Here's how the part is built. I have some questions about the finished solid (model axes, mm). Face numbers are marked on the shaded views. Coordinates: 2 decimals unless noted, no trailing zeros. Loops run counter-clockwise (first coordinate to the right, second up) from the corner with the lowest first, then second, coordinate; pieces in that order, holes last. Notation, with made-up numbers: M 33,36.25 L 67,36.25 A27 ccw 67,55.25 Z; hole C 62,25.25 d7. An arc over 180 degrees is marked long. Use CSV: the item, a comma, the result in double quotes. Start each with the question number.
Q1. For pin 1 Ø8 at (x, y) = (-20.5, 55.5) entering from -Z; pin 2 Ø10.5 at (x, z) = (-53, -18.5) entering from -Y; pin 3 Ø3 at (x, y) = (-41, 46) entering from +Z; pin 4 Ø3 at (x, z) = (-47, 41.5) entering from -Y, each with a flat end and sliding along its axis, tell me the tip position at first contact or that it passes through.
Q2. If we section it at C-C (z = 44): Please give me the cut outline in (x, y).
Q3. If we section it at B-B (x = -44): State how many separate pieces and enclosed holes the cut face has, and give its area (3 significant figures).
Q4. If we mould it in two halves opening along Z, with no side actions, what happens to the marked faces 1, 2, 3 and 4? For each: +Z half, -Z half, draft (parallel to the pull), parting line (faces both ways), or undercut.
Q5. If we section it at A-A (z = 68): Please give me the cut outline in (x, y).
Q6. Please list where these lines run through material, in increasing order: probe 1 along Y at (x, z) = (-40, 65); probe 2 along X at (y, z) = (7, 12); probe 3 along Z at (x, y) = (-22.5, 64). Write a range as [from, to].
Q7. If we section it at D-D (y = 53): Please give me the cut outline in (x, z).
from build123d import *

# Parameters (mm, degrees)
F0_W      = 76
F0_H      = 76
F0_W_2    = 68
F0_H_2    = 68
F1_DEPTH  = 100
F2_W      = 68
F2_H      = 4
F3_DEPTH  = 25
F5_DEPTH  = 72
F7_DEPTH  = 76
F9_DEPTH  = 25
F11_DEPTH = 72


with BuildPart() as f1:
    # F0 (on Top) → F1 (new body)
    with BuildSketch(Plane.XY):
        with Locations((-38, 38)):
            Rectangle(F0_W, F0_H)
        with Locations((-38, 38)):
            Rectangle(F0_W_2, F0_H_2, mode=Mode.SUBTRACT)
    extrude(amount=F1_DEPTH)

    # F2 (on face) → F3 (join)
    with BuildSketch(Plane.XY):
        Polygon((-76, 76), (-76, 0), (-72, 0), (-72, 72), (-72, 76), align=None)
        with Locations((-38, 74)):
            Rectangle(F2_W, F2_H)
        Polygon((-4, 76), (-4, 72), (-4, 0), (0, 0), (0, 76), align=None)
    extrude(amount=-F3_DEPTH)

    # F4 (on face) → F5 (join, through all)
    with BuildSketch(Plane(origin=(-76, 0, 0), x_dir=(0, -1, 0), z_dir=(-1, 0, 0))):
        Polygon((-10.85203, -25), (-71.971662, 0), (-76, 0), (-76, -2.726357), (-21.37715, -25), align=None)
    extrude(amount=-F5_DEPTH)

    # F6 (on face) → F7 (cut, through all)
    with BuildSketch(Plane(origin=(-76, 0, 0), x_dir=(0, -1, 0), z_dir=(-1, 0, 0))):
        with BuildLine():
            Line((0, -25), (0, 0))
            ThreePointArc((0, 0), (-9.849808, -7.286393), (-12.617335, -19.221678))
            Line((-12.617335, -19.221678), (0, -25))
        make_face()
    extrude(amount=-F7_DEPTH, mode=Mode.SUBTRACT)

    # F8 (on face) → F9 (cut)
    with BuildSketch(Plane.XZ):
        with BuildLine():
            Line((-72, 0), (-4, 0))
            ThreePointArc((-4, 0), (-38, 9.360839), (-72, 0))
        make_face()
    extrude(amount=-F9_DEPTH, mode=Mode.SUBTRACT)

    # F10 (on face) → F11 (join, through all)
    with BuildSketch(Plane(origin=(-76, 0, 0), x_dir=(0, -1, 0), z_dir=(-1, 0, 0))):
        Polygon((-37.44344, 15.143791), (-37.44344, 11.143791), (0, 25.214639), (0, 29.214639), align=None)
        Polygon((-71.970133, 51.007654), (-40.531019, 36.690459), (-40.531019, 40.690459), (-71.970133, 55.007654), align=None)
    extrude(amount=-F11_DEPTH)


solid = f1.part
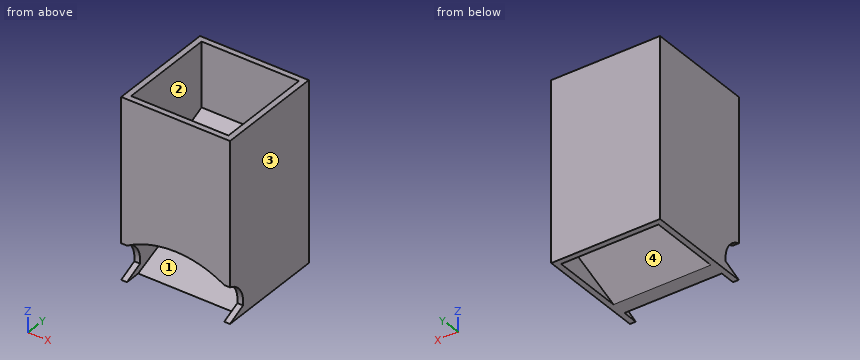
Results below:
1,pin 1,"z = -12.72"
1,pin 2,"y = 13.91"
1,pin 3,"z = 43.86"
1,pin 4,"y = 0"
2,outline,"M -76,0 L 0,0 L 0,76 L -76,76 Z; hole M -72,4 L -4,4 L -4,47.8 L -72,47.8 Z; hole M -72,56.58 L -4,56.58 L -4,72 L -72,72 Z"
3,separate pieces,"3"
3,enclosed holes,"0"
3,area,"1,370 mm^2"
4,face 1,"undercut"
4,face 2,"undercut"
4,face 3,"draft"
4,face 4,"-Z half"
5,outline,"M -76,0 L 0,0 L 0,76 L -76,76 Z; hole M -72,4 L -4,4 L -4,72 L -72,72 Z"
6,probe 1,"[0, 4], [72, 76]"
6,probe 2,"[-76, -72], [-4, 0]"
6,probe 3,"[-7.62, -3.26], [47.38, 51.38]"
7,outline,"M -76,-25 L -72,-25 L -72,-12.11 L -4,-12.11 L -4,-25 L 0,-25 L 0,100 L -4,100 L -4,46.37 L -72,46.37 L -72,100 L -76,100 Z; hole M -72,-7.76 L -4,-7.76 L -4,42.37 L -72,42.37 Z"
